```python
from build123d import *

# Parameters (mm, degrees)
EXTRUDE_THIN1_DEPTH = 5


with BuildPart() as part:
    # Sketch1 → Extrude-Thin1 (new, symmetric)
    with BuildSketch(Plane(origin=(0, 0, 0), x_dir=(0, 0, -1), z_dir=(1, 0, 0))):
        with BuildLine():
            Line((-77.503218133, 17.000038263), (-637.553569857, 14.999904342))
            ThreePointArc((-637.553569857, 14.999904342), (-652.499976085, -0.026784971), (-637.5, -15))
            Line((-637.5, -15), (637.5, -15))
            ThreePointArc((637.5, -15), (652.499983614, -0.022171887), (637.544343726, 14.999934454))
            Line((637.544343726, 14.999934454), (-39.020955624, 17.000038263))
            ThreePointArc((-39.020955624, 17.000038263), (-43.252125342, 18.763647149), (-45.003218133, 23.000012045))
            Line((-45.003218133, 23.000012045), (-45.003218133, 32.000038263))
            Line((-45.003218133, 32.000038263), (-43.503218133, 32.000038263))
            Line((-43.503218133, 32.000038263), (-43.503218133, 23.000012045))
            ThreePointArc((-43.503218133, 23.000012045), (-42.18989854, 19.822738373), (-39.016521251, 18.500031709))
            Line((-39.016521251, 18.500031709), (637.548778098, 16.4999279))
            ThreePointArc((637.548778098, 16.4999279), (653.999981975, -0.024389076), (637.5, -16.5))
            Line((637.5, -16.5), (-637.5, -16.5))
            ThreePointArc((-637.5, -16.5), (-653.999973694, -0.029463469), (-637.558926843, 16.499894776))
            Line((-637.558926843, 16.499894776), (-77.508575119, 18.500028697))
            Line((-77.508575119, 18.500028697), (-77.503218133, 17.000038263))
        make_face()
    extrude(amount=EXTRUDE_THIN1_DEPTH, both=True)


solid = part.part
```
The model under review builds one solid part; all positions refer to its coordinate system, in mm. Coordinates: 2 decimals unless noted, no trailing zeros. Loops run counter-clockwise (first coordinate to the right, second up) from the corner with the lowest first, then second, coordinate; pieces in that order, holes last. Notation, with made-up numbers: (61.25, 55.25) -> (118.25, 55.25) arc R37 ccw to (118.25, 93.25) -> close; hole circle Ø8 at (54.25, 7). An arc over 180 degrees is marked (long way). Answer as CSV lines item,"result".
Item 1: For L1, parallel to Y at x = -4.25, z = 83.5; L2, parallel to Y at x = -3.25, z = 111.5; L3, parallel to Z at x = 0.75, y = 9, list the stretches that pass through material, from the lowest coordinate up.
Results below:
L1,"y = -16.5 to -15, 16.98 to 18.48"
L2,"y = -16.5 to -15, 16.88 to 18.38"
L3,"z = -651.33 to -649.5, 649.5 to 651.33"
Item 2: Take a section at A-A, the plane y = 0. State the section outline as (x, z) points.
Results below:
outline,"(-5, -654) -> (5, -654) -> (5, -652.5) -> (-5, -652.5) -> close; (-5, 652.5) -> (5, 652.5) -> (5, 654) -> (-5, 654) -> close"
Item 3: Draft analysis for pull direction X (two halves, no side actions). For faces 1 (the flat face through (5, -15.5, -3.1)), 2 (the flat face through (-5, -15.5, -3.1)), state which applies: +X half, -X half, draft (parallel to the pull), parting line (faces both ways), or undercut.
Results below:
face 1,"+X half"
face 2,"-X half"
Item 4: Take a section at C-C, the plane z = -562.5. State the section outline as (x, y) points, and give its area (3 significant figures).
Results below:
outline,"(-5, -16.5) -> (5, -16.5) -> (5, -15) -> (-5, -15) -> close; (-5, 15.22) -> (5, 15.22) -> (5, 16.72) -> (-5, 16.72) -> close"
area,"30.0 mm2"
Item 5: Insertion check: pin 1 (1.5 mm diameter, centred on x = -1, y = -3.5, fed in from -Z); pin 2 (6 mm diameter, centred on y = -11.5, z = 142, fed in from +X) (3 decimals); pin 3 (2.5 mm diameter, centred on x = -2, y = 27.5, fed in from -Z). Each pin has a flat end and moves straight along its axis. Give the tip position at first contact, or say it passes through.
Results below:
pin 1,"stops at z = -653.77"
pin 2,"passes through"
pin 3,"stops at z = 43.5"
Item 6: Take a section at B-B, the plane x = 0. State the section outline as (y, z) points, and give its area (3 significant figures).
Results below:
outline,"(-16.5, -637.5) arc R16.5 ccw to (16.5, -637.55) -> (18.5, 39.02) arc R4.5 cw to (23, 43.5) -> (32, 43.5) -> (32, 45) -> (23, 45) arc R6 ccw to (17, 39.02) -> (15, -637.54) arc R15 cw to (-15, -637.5) -> (-15, 637.5) arc R15 cw to (15, 637.55) -> (17, 77.5) -> (18.5, 77.51) -> (16.5, 637.56) arc R16.5 ccw to (-16.5, 637.5) -> close"
area,"3,940 mm2"
